Autodesk Inventor part; units mm, degrees
ref_plane "Work Plane1" through (0, 12, 0) normal (0, 1, 0) x (-1, 0, 0)
ref_plane "YZ Plane" through (0, 0, 0) normal (1, 0, 0) x (0, 1, 0)
ref_plane "XY Plane" through (0, 0, 0) normal (0, 0, 1) x (1, 0, 0)
sketch "Sketch1" plane through (0, 0, 0) normal (1, 0, 0) x (0, 1, 0)
  circle A0 centre (0, 0) radius 12
  dimension "d0" = 24
extrude "Extrusion1" add sketch "Sketch1" along normal blind 34
chamfer "Chamfer1" distance 2 angle 45 1 edges at (34, -12, 0)
sketch "Sketch2" plane through (0, 0, 0) normal (0, 0, 1) x (1, 0, 0)
  line L0 (0, -12) -> (0, 12) construction
  line L1 (32, -12) -> (32, 12) construction
  line L2 (0, 0) -> (32, 0) construction
  line L3 (14, 5) -> (34, 5)
  line L4 (34, -5) -> (14, -5)
  line L5 (34, 10) -> (34, -10)
  arc A0 (14, 5) -> (14, -5) centre (14, 0) ccw
  dimension "d8" = 10
  dimension "d9" = 5
extrude "Extrusion2" cut sketch "Sketch2" along normal through all both and the other way through all
sketch "Sketch5" plane through (0, 0, 0) normal (1, 0, 0) x (0, 1, 0)
  circle A0 centre (0, 0) radius 12 construction
  circle A1 centre (0, 0) radius 6
  dimension "d27" = 12
extrude "Extrusion3" add sketch "Sketch5" against normal blind 8
sketch "Sketch6" plane through (-8, 0, 0) normal (-1, 0, 0) x (0, 0, 1)
  circle A0 centre (0, 0) radius 6
  circle A1 centre (0, 0) radius 8
  dimension "d30" = 16
extrude "Extrusion4" add sketch "Sketch6" along normal blind 18 contours A0 | A1
fillet "Fillet1" radius 2 2 edges at (0, -6, 0) (-8, -6, 0)
chamfer "Chamfer2" distance 1 angle 45 1 edges at (-26, 0, -8)
sketch "Sketch7" plane through (-26, 0, 0) normal (-1, 0, 0) x (0, 0, 1)
  circle A0 centre (0, 0) radius 8
hole "Hole3" at (-26, 0, 0) direction (1, 0, 0) diameter 6.647 depth 22.2 tip angle 118
ref_plane "Work Plane1" through (0, 12, 0) normal (0, 1, 0) x (-1, 0, 0)
sketch "Sketch9" plane through (0, 12, 0) normal (0, 1, 0) x (-1, 0, 0)
  line L0 (0, 12) -> (0, -12) construction
  line L1 (-32, 10.9087) -> (-14, 10.9087) construction
  line L2 (-14, 10.9087) -> (-32, 10.9087) construction
  line L3 (-32, -10.9087) -> (-32, 10.9087) construction
  line L4 (-32, -10.9087) -> (-14, -10.9087) construction
  line L5 (-14, -10.9087) -> (-32, -10.9087) construction
  line L6 (-32, 10.9087) -> (-32, -10.9087) construction
  line L7 (-34, -8.6603) -> (-34, 8.6603) construction
  point P0 (0, 0)
  point P1 (-24, 0)
  point P2 (-34, 0)
  dimension "d52" = 10
hole "Hole5" at (24, 12, 0) direction (0, -1, 0) diameter 8.376 depth 27.3 tip angle 118
properties part number "Part11.End Fork" material "Steel, Carbon"
Check sheet for the modelled part. Datum: model origin and axes. Units: mm. A direction names the side the tool comes from. Coordinates: 2 decimals unless noted, no trailing zeros. Loops run counter-clockwise (first coordinate to the right, second up) from the corner with the lowest first, then second, coordinate; pieces in that order, holes last. Notation, with made-up numbers: (37.25, 48.5) -> (63.25, 48.5) arc R29 cw to (63.25, 83.5) -> close; hole circle Ø9 at (-24, 54.5). An arc over 180 degrees is marked (long way). Write item = value, one per line. Start each with the question number.
1. Section check A-A on x = 24. Record the cut outline in (y, z).
2. Draft check along Z on faces 1 (the cylindrical face through (9, 0, 0)), 2 (the conical face through (33.875, -10.124, -0.162)), 3 (the cylindrical face through (-14.74, 1.27, 3.07)). Enter one of: released by +Z, released by -Z, zero draft, split by the parting line, or undercut.
3. Section check C-C on z = -2. Give the number of separate pieces and of enclosed holes in the cut face, then the cut area to 3 significant figures.
4. Tool access check on faces 4 (the cylindrical face through (-16.38, 7.81, -1.73)), 5 (the cylindrical face through (-4, -6, 0)), 6 (the flat face through (34, -7, 0)), 7 (the flat face through (19, 5, 0)). Record the directions out of +Z, -Z, +X, -X, +Y, -Y that give a thin tool (end or side, any length) a straight path to the whole face; none if there is none.
5. Depth check by flat-ended pin: P1, Ø3, axis at y = -9.5, z = -5.5, coming from the -X side; P2, Ø10, axis at x = -8, z = -7.5, coming from the -Y side; P3, Ø2, axis at x = 3.5, z = -8.5, coming from the -Y side; P4, Ø7.5, axis at x = 24, z = 0, coming from the -Y side. Enter the tip coordinate at first touch or a pass-through.
6. Material ranges on line 1 (X direction, y = 7.25, z = 0); line 2 (Y direction, x = -12.5, z = 0); line 3 (X direction, y = 8.25, z = 0), recorded low to high.
7. Section check B-B on x = -12.5. Record the cut outline in (y, z), then the cut area to 3 significant figures.
Responses:
q1.outline = (-11.25, -4.19) arc R12 ccw to (-5, -10.91) -> (-5, -4.19) -> close; (-11.25, 4.19) -> (-5, 4.19) -> (-5, 10.91) arc R12 ccw to start; (5, -10.91) arc R12 ccw to (11.25, -4.19) -> (5, -4.19) -> close; (5, 4.19) -> (11.25, 4.19) arc R12 ccw to (5, 10.91) -> close
q2.face_1 = zero draft
q2.face_2 = split by the parting line
q2.face_3 = undercut
q3.separate_pieces = 3
q3.enclosed_holes = 0
q3.area = 712 mm2
q4.face_4 = -X
q4.face_5 = none
q4.face_6 = +Z, -Z, +X, +Y, -Y
q4.face_7 = +Z, -Z, +X
q5.P1 = 0
q5.P2 = -7.6
q5.P3 = -9.37
q5.P4 = through
q6.line_1 = -25.75 to -7.85, -0.15 to 19.81, 28.19 to 34
q6.line_2 = -8 to -3.32, 3.32 to 8
q6.line_3 = 0 to 19.81, 28.19 to 34
q7.outline = circle Ø16 at (0, 0); hole circle Ø6.65 at (0, 0)
q7.area = 166 mm2
